For this review, use the dimensioned drawing (mm, ordinates from the lowest corner) and the shaded views. A direction names the side the tool comes from. Coordinates: 2 decimals unless noted, no trailing zeros. Write each loop counter-clockwise with the first axis right and the second up, starting at its lowest first coordinate (ties: lowest second). Pieces come first, ordered by that corner, then holes. Notation, with made-up numbers: M 20.25,71 L 74.25,71 A16 ccw 74.25,85 Z; hole C -24.75,-6 d9. An arc over 180 degrees is marked long. Return JSON: item names as keys, results as strings. Group by question number.
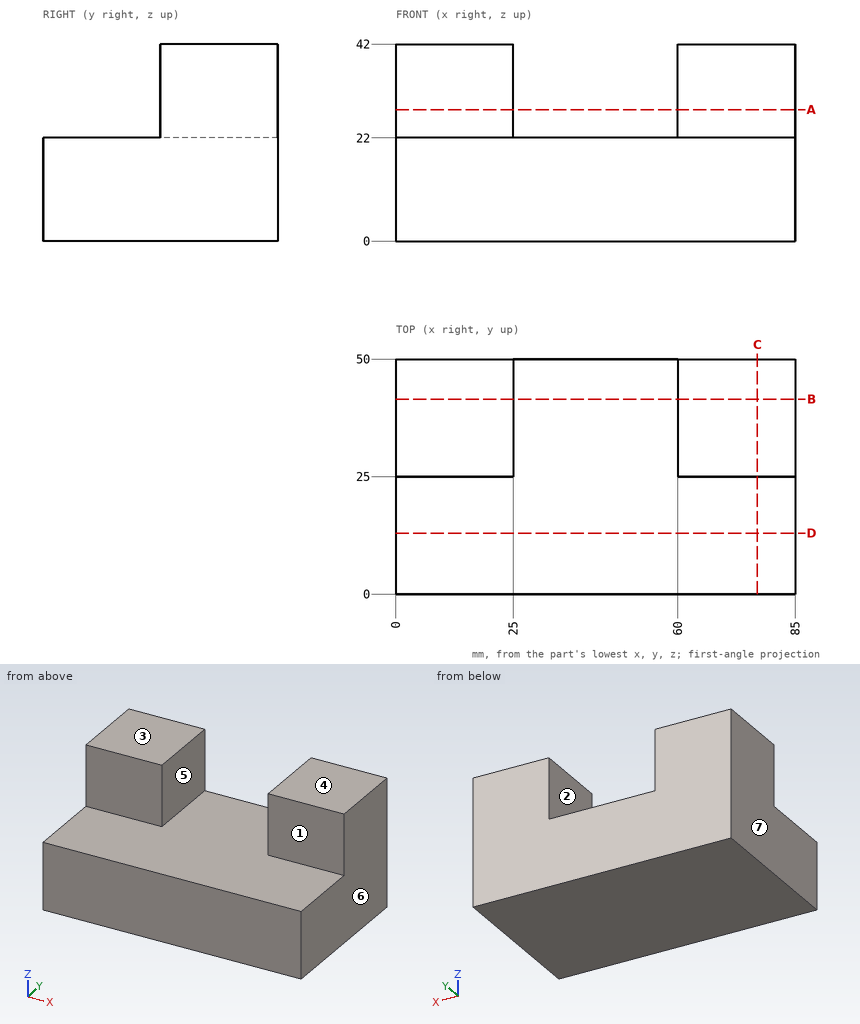
Item 1: Add section C-C (x = 77). Write out the cut boundary in (y, z).
Item 2: The part is to be moulded in two halves that separate along X. For the marked faces 4, 5, 6 and 7, say which applies: pulls with the +X half, pulls with the -X half, needs draft (parallel to the pull), parting line crosses it, or undercut.
Item 3: Add section D-D (y = 13). Write out the cut boundary in (x, z), plus the area to 3 significant figures.
Item 4: For pin 1 (6 mm diameter, centred on y = 44.5, z = 32, fed in from -X); pin 2 (3 mm diameter, centred on x = 18.5, y = 19, fed in from +Z); pin 3 (6 mm diameter, centred on x = 72, z = 37, fed in from -Y), all flat-tipped, find the tip position at first contact; note any pin that passes through.
Item 5: Add section B-B (y = 41.5). Write out the cut boundary in (x, z).
Item 6: Add section A-A (z = 28). Write out the cut boundary in (x, y), plus the area to 3 significant figures.
Item 7: For line 1 (X direction, y = 36.5, z = 26.5); line 2 (Z direction, x = 51, y = 35); line 3 (Y direction, x = 80.5, z = 24), list the stretches that pass through material, from the lowest coordinate up.
Item 8: Machinability: for the marked faces 1, 2 and 3, which of the approach directions +Z, -Z, +X, -X, +Y, -Y give a long, thin tool a straight path to every point of the face, cutting with its end or side? Answer none if there is none.
Geometry check:
{
 "1": {"outline": "M 0,0 L 50,0 L 50,42 L 25,42 L 25,22 L 0,22 Z"},
 "2": {"face 4": "needs draft", "face 5": "undercut", "face 6": "pulls with the +X half", "face 7": "pulls with the -X half"},
 "3": {"outline": "M 0,0 L 85,0 L 85,22 L 0,22 Z", "area": "1,870 mm^2"},
 "4": {"pin 1": "x = 0", "pin 2": "z = 22", "pin 3": "y = 25"},
 "5": {"outline": "M 0,0 L 85,0 L 85,42 L 60,42 L 60,22 L 25,22 L 25,42 L 0,42 Z"},
 "6": {"outline": "M 0,25 L 25,25 L 25,50 L 0,50 Z; M 60,25 L 85,25 L 85,50 L 60,50 Z", "area": "1,250 mm^2"},
 "7": {"line 1": "0 to 25, 60 to 85", "line 2": "0 to 22", "line 3": "25 to 50"},
 "8": {"face 1": "+Z, +X, -X, -Y", "face 2": "+Z, +Y, -Y", "face 3": "+Z, +X, -X, +Y, -Y"}
}
